Design review of the part built by this model. Coordinates are the model's own, in mm. A direction names the side the tool comes from. Coordinates: 2 decimals unless noted, no trailing zeros. Loops run counter-clockwise (first coordinate to the right, second up) from the corner with the lowest first, then second, coordinate; pieces in that order, holes last. Notation, with made-up numbers: M -22,67.25 L -8,67.25 A34 cw -8,101.25 Z; hole C 19,59.25 d11. An arc over 180 degrees is marked long. Answer as a JSON object with one key per item and string values. Group by question number.
1. Machinability: for faces 1 (the flat face through (3, 6.5, -5)), 2 (the flat face through (3, -5, 6.5)), 3 (the flat face through (3, -5.5, -4)), 4 (the cylindrical face through (24.1, -4.05, 0.9)), 5 (the flat face through (3, 2, 8)), which of the approach directions +Z, -Z, +X, -X, +Y, -Y give a long, thin tool a straight path to every point of the face, cutting with its end or side? Answer none if there is none.
2. Consider section C-C (x = 10.5). State the section outline as (y, z) points.
3. Consider section D-D (y = 8.75). State the section outline as (x, z) points, then the cut area to 3 significant figures.
4. Insertion check: pin 1 (1 mm diameter, centred on y = -0.5, z = -4, fed in from -X); pin 2 (5 mm diameter, centred on x = 13.5, z = 10.5, fed in from +Y); pin 3 (1 mm diameter, centred on x = 3.5, z = 5.5, fed in from -Y); pin 4 (1 mm diameter, centred on x = 3, z = 4, fed in from +Y). Each pin has a flat end and moves straight along its axis. Give the tip position at first contact, or say it passes through.
5. To check wall thickness, follow probe 1 along X at (y, z) = (3.5, 4.25); probe 2 along X at (y, z) = (-4.25, -4.5); probe 3 along Y at (x, z) = (23.05, 0). State the ranges of each line that lie inside material, in increasing order.
6. Draft analysis for pull direction X (two halves, no side actions). For faces 6 (the cylindrical face through (21.583, 5.773, -2.394)), 7 (the flat face through (5.1, -5.4, 5.4)), 8 (the flat face through (1, 0, -15)), state which applies: +X half, -X half, draft (parallel to the pull), parting line (faces both ways), or undercut.
7. Consider section B-B (z = -12). State the section outline as (x, y) points, then the cut area to 3 significant figures.
8. Consider section A-A (x = 4.5). State the section outline as (y, z) points, then the cut area to 3 significant figures.
from build123d import *

# Parameters (mm, degrees)
CROQUIS_BASE_W               = 30
CROQUIS_BASE_H               = 24
PLACA_ELECTRONICA_DEPTH      = 1.6
CORTAR_EXTRUIR3_DEPTH        = 20.275891678
CROQUIS_MONTAJE_CAMARA_R     = 0.75
SALIENTE_EXTRUIR2_DEPTH      = 3.5
SALIENTE_EXTRUIR3_DEPTH      = 8.75
SALIENTE_EXTRUIR3_DEPTH_BACK = 3.5
CAMERA_STAGE_1_R             = 7
CAMERA_STAGE_2_R             = 5.875
SALIENTE_EXTRUIR4_DEPTH      = 5.5
SALIENTE_EXTRUIR5_START      = 5
CAMERA_STAGE_3_R             = 7
SALIENTE_EXTRUIR5_DEPTH      = 5
VACIADO5_START               = 1
VACIADO5_OUTLINE_R           = 5.125
VACIADO5_DEPTH               = 23.35
VACIADO5_2_OUTLINE_R         = 6
VACIADO5_2_OUTLINE_R_2       = 5.125
VACIADO5_2_DEPTH             = 11.85
VACIADO5_START_2             = 20.35
VACIADO5_3_OUTLINE_R         = 6.25
VACIADO5_3_OUTLINE_R_2       = 5.125
VACIADO5_3_DEPTH             = 4
VACIADO5_4_DEPTH             = 3.1
SALIENTE_EXTRUIR6_START      = -1.5
CROQUIS_LENTE_R              = 6.25
SALIENTE_EXTRUIR6_DEPTH      = 1.5
CROQUIS_LENTE_3_R            = 4.15
CORTAR_EXTRUIR2_DEPTH        = 1.5
SALIENTE_EXTRUIR7_START      = 0.5
CROQUIS_DEL_LENTE_R          = 4.15
SALIENTE_EXTRUIR7_DEPTH      = 0.5


# Read off the part's stored shape, not the designer's step: Vaciado5
with BuildPart() as part:
    # Croquis base → Placa electronica (new body)
    with BuildSketch(Plane(origin=(0, 0, 0), x_dir=(0, 0, -1), z_dir=(1, 0, 0))):
        Rectangle(CROQUIS_BASE_W, CROQUIS_BASE_H)
    extrude(amount=PLACA_ELECTRONICA_DEPTH)

    # Croquis barrenos → Cortar-Extruir3 (cut, through all)
    with BuildSketch(Plane(origin=(1.6, 0, 0), x_dir=(0, 0, -1), z_dir=(1, 0, 0))):
        with BuildLine():
            Line((-13.25, 12), (-10.75, 12))
            ThreePointArc((-10.75, 12), (-12, 10.75), (-13.25, 12))
        make_face()
        with BuildLine():
            Line((-13.25, -12), (-10.75, -12))
            ThreePointArc((-10.75, -12), (-12, -10.75), (-13.25, -12))
        make_face()
        with BuildLine():
            Line((10.75, 12), (13.25, 12))
            ThreePointArc((13.25, 12), (12, 10.75), (10.75, 12))
        make_face()
        with BuildLine():
            Line((10.75, -12), (13.25, -12))
            ThreePointArc((13.25, -12), (12, -10.75), (10.75, -12))
        make_face()
    extrude(amount=-CORTAR_EXTRUIR3_DEPTH, mode=Mode.SUBTRACT)

    # Croquis montaje camara → Saliente-Extruir2 (add)
    with BuildSketch(Plane(origin=(1.6, 0, 0), x_dir=(0, 0, -1), z_dir=(1, 0, 0))):
        with BuildLine():
            Line((-6.5, 6.5), (6.5, 6.5))
            Line((6.5, 6.5), (6.5, 2))
            Line((6.5, 2), (8.5, 2))
            ThreePointArc((8.5, 2), (10.5, 0), (8.5, -2))
            Line((8.5, -2), (6.5, -2))
            Line((6.5, -2), (6.5, -6.5))
            Line((6.5, -6.5), (-6.5, -6.5))
            Line((-6.5, -6.5), (-6.5, -2))
            Line((-6.5, -2), (-8.5, -2))
            ThreePointArc((-8.5, -2), (-10.5, 0), (-8.5, 2))
            Line((-8.5, 2), (-6.5, 2))
            Line((-6.5, 2), (-6.5, 6.5))
        make_face()
        with Locations((-8.5, 0)):
            Circle(CROQUIS_MONTAJE_CAMARA_R, mode=Mode.SUBTRACT)
        with Locations((8.5, 0)):
            Circle(CROQUIS_MONTAJE_CAMARA_R, mode=Mode.SUBTRACT)
    extrude(amount=SALIENTE_EXTRUIR2_DEPTH)

    # Camera Stage 1 → Saliente-Extruir3 (add, two sides: drawn at the far end of the back side and taken through both)
    with BuildSketch(Plane(origin=(5.1, 0, 0), x_dir=(0, 0, -1), z_dir=(1, 0, 0)).offset(-SALIENTE_EXTRUIR3_DEPTH_BACK)):
        Circle(CAMERA_STAGE_1_R)
    extrude(amount=SALIENTE_EXTRUIR3_DEPTH + SALIENTE_EXTRUIR3_DEPTH_BACK)

    # Camera Stage 2 → Saliente-Extruir4 (add)
    with BuildSketch(Plane(origin=(13.85, 0, 0), x_dir=(0, 0, -1), z_dir=(1, 0, 0))):
        Circle(CAMERA_STAGE_2_R)
    extrude(amount=SALIENTE_EXTRUIR4_DEPTH)

    # Camera Stage 3 → Saliente-Extruir5 (add)
    with BuildSketch(Plane(origin=(19.35, 0, 0), x_dir=(0, 0, -1), z_dir=(1, 0, 0)).offset(SALIENTE_EXTRUIR5_START)):
        Circle(CAMERA_STAGE_3_R)
    extrude(amount=-SALIENTE_EXTRUIR5_DEPTH)

    # Vaciado5 outline → Vaciado5 (cut)
    with BuildSketch(Plane.YZ.offset(VACIADO5_START)):
        Circle(VACIADO5_OUTLINE_R)
    extrude(amount=VACIADO5_DEPTH, mode=Mode.SUBTRACT)

    # Vaciado5 2 outline → Vaciado5 2 (cut)
    with BuildSketch(Plane.YZ.offset(VACIADO5_START)):
        Circle(VACIADO5_2_OUTLINE_R)
        Circle(VACIADO5_2_OUTLINE_R_2, mode=Mode.SUBTRACT)
    extrude(amount=VACIADO5_2_DEPTH, mode=Mode.SUBTRACT)

    # Vaciado5 3 outline → Vaciado5 3 (cut)
    with BuildSketch(Plane.YZ.offset(VACIADO5_START_2)):
        Circle(VACIADO5_3_OUTLINE_R)
        Circle(VACIADO5_3_OUTLINE_R_2, mode=Mode.SUBTRACT)
    extrude(amount=VACIADO5_3_DEPTH, mode=Mode.SUBTRACT)

    # Vaciado5 4 outline → Vaciado5 4 (cut)
    with BuildSketch(Plane.YZ.offset(VACIADO5_START)):
        with BuildLine():
            ThreePointArc((-1, 5.916079783), (0, 6), (1, 5.916079783))
            Line((1, 5.916079783), (1, 7.063859338))
            ThreePointArc((1, 7.063859338), (0, 6.75), (-1, 7.063859338))
            Line((-1, 7.063859338), (-1, 5.916079783))
        make_face()
        with BuildLine():
            ThreePointArc((-5.5, 2.397915762), (-4.242640687, 4.242640687), (-2.397915762, 5.5))
            Line((-2.397915762, 5.5), (-5.5, 5.5))
            Line((-5.5, 5.5), (-5.5, 2.397915762))
        make_face()
        with BuildLine():
            ThreePointArc((2.397915762, 5.5), (4.242640687, 4.242640687), (5.5, 2.397915762))
            Line((5.5, 2.397915762), (5.5, 5.5))
            Line((5.5, 5.5), (2.397915762, 5.5))
        make_face()
        with BuildLine():
            ThreePointArc((-2.397915762, -5.5), (-4.242640687, -4.242640687), (-5.5, -2.397915762))
            Line((-5.5, -2.397915762), (-5.5, -5.5))
            Line((-5.5, -5.5), (-2.397915762, -5.5))
        make_face()
        with BuildLine():
            ThreePointArc((5.5, -2.397915762), (4.242640687, -4.242640687), (2.397915762, -5.5))
            Line((2.397915762, -5.5), (5.5, -5.5))
            Line((5.5, -5.5), (5.5, -2.397915762))
        make_face()
        with BuildLine():
            ThreePointArc((1, -5.916079783), (0, -6), (-1, -5.916079783))
            Line((-1, -5.916079783), (-1, -7.063859338))
            ThreePointArc((-1, -7.063859338), (0, -6.75), (1, -7.063859338))
            Line((1, -7.063859338), (1, -5.916079783))
        make_face()
    extrude(amount=VACIADO5_4_DEPTH, mode=Mode.SUBTRACT)

    # Croquis lente → Saliente-Extruir6 (add)
    with BuildSketch(Plane(origin=(24.35, 0, 0), x_dir=(0, 0, -1), z_dir=(1, 0, 0)).offset(SALIENTE_EXTRUIR6_START)):
        Circle(CROQUIS_LENTE_R)
    extrude(amount=SALIENTE_EXTRUIR6_DEPTH)

    # Croquis lente<3> → Cortar-Extruir2 (cut)
    with BuildSketch(Plane(origin=(24.35, 0, 0), x_dir=(0, 0, -1), z_dir=(1, 0, 0))):
        Circle(CROQUIS_LENTE_3_R)
    extrude(amount=-CORTAR_EXTRUIR2_DEPTH, mode=Mode.SUBTRACT)

    # Croquis del lente → Saliente-Extruir7 (add)
    with BuildSketch(Plane(origin=(23.35, 0, 0), x_dir=(0, 0, -1), z_dir=(1, 0, 0)).offset(SALIENTE_EXTRUIR7_START)):
        Circle(CROQUIS_DEL_LENTE_R)
    extrude(amount=-SALIENTE_EXTRUIR7_DEPTH)


solid = part.part
Findings below:
{
 "1": {"face 1": "-Z, +X, +Y", "face 2": "+Z, +X, -Y", "face 3": "none", "face 4": "+X", "face 5": "+Z, +X, +Y"},
 "2": {"outline": "C 0,0 d14; hole C 0,0 d12"},
 "3": {"outline": "M 0,-15 L 1.6,-15 L 1.6,15 L 0,15 Z", "area": "48.0 mm^2"},
 "4": {"pin 1": "stops at x = 0", "pin 2": "passes through", "pin 3": "stops at y = -6.5", "pin 4": "stops at y = 6.5"},
 "5": {"probe 1": "x = 0 to 1, 12.85 to 20.35, 22.85 to 24.35", "probe 2": "x = 0 to 1, 4.1 to 13.85, 19.35 to 20.35, 22.85 to 24.35", "probe 3": "y = -7 to -4.15, 4.15 to 7"},
 "6": {"face 6": "undercut", "face 7": "+X half", "face 8": "draft"},
 "7": {"outline": "M 0,-10.75 L 1.6,-10.75 L 1.6,10.75 L 0,10.75 Z", "area": "34.4 mm^2"},
 "8": {"outline": "M -6.5,-6.5 L -2.6,-6.5 A7 ccw -2,-6.71 L -2,-8.5 A2 ccw 2,-8.5 L 2,-6.71 A7 ccw 2.6,-6.5 L 6.5,-6.5 L 6.5,-2.6 A7 ccw 6.5,2.6 L 6.5,6.5 L 2.6,6.5 A7 ccw 2,6.71 L 2,8.5 A2 ccw -2,8.5 L -2,6.71 A7 ccw -2.6,6.5 L -6.5,6.5 L -6.5,2.6 A7 ccw -6.5,-2.6 Z; hole C 0,0 d12; hole C 0,-8.5 d1.5; hole C 0,8.5 d1.5", "area": "84.7 mm^2"}
}
